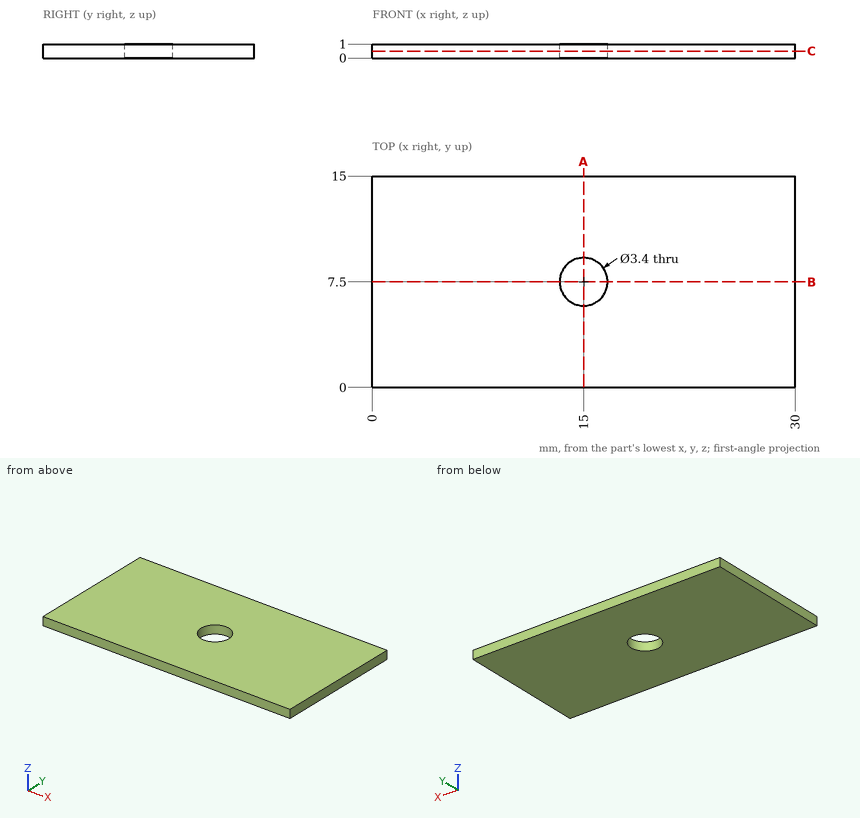
Study the drawing (mm; zero at the part's minimum x, y, z) and answer. Round coordinates to 2 decimals unless told otherwise and drop trailing zeros. Order: outer loops, then holes, each group sorted by start corner. A loop starts at its lowest first (then second) coordinate and runs counter-clockwise, first axis right, second up. Notation, with made-up numbers: (52.25, 16) - (61.25, 16) arc R18 ccw to (61.25, 27) - close; hole circle Ø7 at (30.5, 22.25). An arc over 180 degrees is marked (long way). Use one line per item in the form item = value. Start each with the question number.
(1) The part is cut by section A-A (x = 15). Give the vertices of the cut face in (y, z), then the cut area to 3 significant figures.
(2) The part is cut by section B-B (y = 7.5). Give the vertices of the cut face in (x, z).
(3) Find the intervals of material crossed by line 1 along X through (y, z) = (9, 0.1); line 2 along X through (y, z) = (7.25, 0.9), in increasing order. Write a range as from..to.
(4) The part is cut by section C-C (z = 0.5). Give the vertices of the cut face in (x, y).
Checked values:
q1.outline = (0, 0) - (5.8, 0) - (5.8, 1) - (0, 1) - close; (9.2, 0) - (15, 0) - (15, 1) - (9.2, 1) - close
q1.area = 11.6 mm^2
q2.outline = (0, 0) - (13.3, 0) - (13.3, 1) - (0, 1) - close; (16.7, 0) - (30, 0) - (30, 1) - (16.7, 1) - close
q3.line_1 = 0..14.2, 15.8..30
q3.line_2 = 0..13.32, 16.68..30
q4.outline = (0, 0) - (30, 0) - (30, 15) - (0, 15) - close; hole circle Ø3.4 at (15, 7.5)
